Source: CAD feature listing. Evaluate the final solid. Frame: model axes, mm. A direction names the side the tool comes from. Coordinates: 2 decimals unless noted, no trailing zeros. Loops run counter-clockwise (first coordinate to the right, second up) from the corner with the lowest first, then second, coordinate; pieces in that order, holes last.
Item 1: Section query D-D, the plane y = 12. Return the cut outline in (x, z).
Item 2: Section query C-C, the plane z = -46.5. Return the cut outline in (x, y).
Item 3: Pin query (flat end, axial travel): pin 1 Ø5.5 at (y, z) = (16.5, 0) entering from +X; pin 2 Ø1.6 at (y, z) = (-1.5, 10.5) entering from -X; pin 3 Ø5 at (x, z) = (8.5, 35) entering from -Y. Return the tip coordinate at first contact, or that it passes through.
Item 4: Section query A-A, the plane z = 30. Return the cut outline in (x, y).
Item 5: Section query B-B, the plane y = 5. Return the cut outline in (x, z), then the cut area to 3 significant figures.
Item 6: Pull-direction query (Y, two-part tool) for faces 1 (the flat face through (1.05, -1, 1)), 2 (the flat face through (3, -2, 1)), 3 (the cylindrical face through (4.791, 12.845, -45.579)); classes: +Y half, -Y half, draft (parallel to the pull), parting line (faces both ways), or undercut.
Item 7: Reachability of faces 4 (the flat face through (3, 0, -50)), 5 (the flat face through (6, 10, -42)), 6 (the flat face through (3, 13, 1)), 7 (the cylindrical face through (1.114, 8.425, -46.563)), 8 (the flat face through (3.95, 4, -50)) from +Z, -Z, +X, -X, +Y, -Y: full face, straight path, thin tool, end or side. Return the list, or none.
Item 8: Line query: probe 1 along Y at (x, z) = (1.3, 0); probe 2 along Z at (x, y) = (7.5, 14.75); probe 3 along Y at (x, z) = (5.25, -8). Output: solid intervals per line, ascending.
```python
from build123d import *

# Parameters (mm, degrees)
MAIN_DEPTH                       = 49
ESQUISSE2_R                      = 1.25
HOLESFORLCDTOP_DEPTH             = 10.45
SKETCH1_W                        = 84
SKETCH1_H                        = 16
POWERBOARDPINHOLES_DEPTH         = 4
SKETCH2_R                        = 1.25
WINDOWFIXHOLES_DEPTH             = 10.45
SKETCH3_W                        = 2.9
SKETCH3_H                        = 20
MAKERBEAMFIX_DEPTH               = 2
SKETCH4_R                        = 1.5
FIXHOLEFORMAKERBEAM_DEPTH        = 20
SKETCH5_W                        = 84
SKETCH5_H                        = 9
HOLESTOHAVEACCESSTOFIXHOLE_DEPTH = 6.45


with BuildPart() as part:
    # Esquisse1 → Main (new body, symmetric)
    with BuildSketch(Plane.XY):
        Polygon((0, 20), (9.45, 20), (9.45, 0), (3.95, 0), (3.95, -2), (1.05, -2), (1.05, 0), (0, 0), align=None)
    extrude(amount=MAIN_DEPTH, both=True)

    # Esquisse2 → HolesForLCDTop (cut, through all)
    with BuildSketch(Plane(origin=(9.45, 0, 0), x_dir=(0, 0, -1), z_dir=(1, 0, 0))):
        with Locations((46.5, 12)):
            Circle(ESQUISSE2_R)
        with Locations((-46.5, 12)):
            Circle(ESQUISSE2_R)
    extrude(amount=-HOLESFORLCDTOP_DEPTH, mode=Mode.SUBTRACT)

    # Sketch1 → PowerBoardPinHoles (cut)
    with BuildSketch(Plane(origin=(9.45, 0, 0), x_dir=(0, 0, -1), z_dir=(1, 0, 0))):
        with Locations((0, 12)):
            Rectangle(SKETCH1_W, SKETCH1_H)
    extrude(amount=-POWERBOARDPINHOLES_DEPTH, mode=Mode.SUBTRACT)

    # Sketch2 → WindowFixHoles (cut, through all)
    with BuildSketch(Plane.ZY):
        with Locations((0, 16.5)):
            Circle(SKETCH2_R)
        with Locations((-30, 16.5)):
            Circle(SKETCH2_R)
        with Locations((30, 16.5)):
            Circle(SKETCH2_R)
    extrude(amount=-WINDOWFIXHOLES_DEPTH, mode=Mode.SUBTRACT)

    # Sketch3 → MakerBeamFix (add)
    with BuildSketch(Plane(origin=(0, 0, -49), x_dir=(-1, 0, 0), z_dir=(0, 0, -1))):
        with Locations((-2.5, 10)):
            Rectangle(SKETCH3_W, SKETCH3_H)
    extrude(amount=MAKERBEAMFIX_DEPTH)

    # Sketch4 → FixHoleForMakerBeam (cut)
    with BuildSketch(Plane(origin=(0, 0, -51), x_dir=(-1, 0, 0), z_dir=(0, 0, -1))):
        with Locations((-2.5, 9)):
            Circle(SKETCH4_R)
    extrude(amount=-FIXHOLEFORMAKERBEAM_DEPTH, mode=Mode.SUBTRACT)

    # Sketch5 → HolesToHaveAccessToFixHole (cut, through all)
    with BuildSketch(Plane(origin=(5.45, 0, 0), x_dir=(0, 0, -1), z_dir=(1, 0, 0))):
        with Locations((0, 8.5)):
            Rectangle(SKETCH5_W, SKETCH5_H)
    extrude(amount=-HOLESTOHAVEACCESSTOFIXHOLE_DEPTH, mode=Mode.SUBTRACT)


solid = part.part
```
Verdict:
1. outline: (0, -49) - (1.05, -49) - (1.05, -51) - (3.95, -51) - (3.95, -49) - (9.45, -49) - (9.45, -47.75) - (0, -47.75) - close; (0, -45.25) - (9.45, -45.25) - (9.45, -42) - (0, -42) - close; (0, 42) - (9.45, 42) - (9.45, 45.25) - (0, 45.25) - close; (0, 47.75) - (9.45, 47.75) - (9.45, 49) - (0, 49) - close
2. outline: (0, 0) - (1.05, 0) - (1.05, -2) - (3.95, -2) - (3.95, 0) - (9.45, 0) - (9.45, 10.75) - (0, 10.75) - close; (0, 13.25) - (9.45, 13.25) - (9.45, 20) - (0, 20) - close; hole circle Ø3 at (2.5, 9)
3. pin 1: stops at x = 5.45
3. pin 2: stops at x = 1.05
3. pin 3: stops at y = 0
4. outline: (0, 0) - (1.05, 0) - (1.05, -2) - (3.95, -2) - (3.95, 0) - (9.45, 0) - (9.45, 4) - (0, 4) - close; (0, 13) - (5.45, 13) - (5.45, 15.25) - (0, 15.25) - close; (0, 17.75) - (5.45, 17.75) - (5.45, 20) - (0, 20) - close
5. outline: (0, -49) - (1.05, -49) - (1.05, -51) - (3.95, -51) - (3.95, -49) - (9.45, -49) - (9.45, -42) - (0, -42) - close; (0, 42) - (9.45, 42) - (9.45, 49) - (0, 49) - close
5. area: 138 mm2
6. face 1: draft
6. face 2: -Y half
6. face 3: undercut
7. face 4: -Z, +X, -X, -Y
7. face 5: +X
7. face 6: +X, -X
7. face 7: -Z
7. face 8: -Z, +X, +Y, -Y
8. probe 1: y = -2 to 4, 13 to 15.25, 17.75 to 20
8. probe 2: z = -49 to -42, 42 to 49
8. probe 3: y = 0 to 4, 13 to 20
